The listing builds one solid part. Answer for the finished solid, in the listing's coordinates (mm). Give positions to 0.01 mm unless a question says otherwise; leave off trailing zeros. Order: outer loops, then holes, each group sorted by start corner. A loop starts at its lowest first (then second) coordinate and runs counter-clockwise, first axis right, second up. Notation, with made-up numbers: (38.5, 86.25) - (62.5, 86.25) arc R15 ccw to (62.5, 91.25) - close; hole circle Ø2 at (43, 23). An arc over 180 degrees is marked (long way). Use a Markdown table: item, result. Add a question column.
1) Flat-ended cylindrical pins translate along their axes: pin 1 (4 mm diameter, centred on x = 84, z = 6.8, fed in from +Y); pin 2 (4 mm diameter, centred on y = -81, z = 44, fed in from +X); pin 3 (1.2 mm diameter, centred on x = -38.5, y = -83, fed in from -Z). Find the tip coordinate at first contact, or state that the pin passes through.
2) Straight lines are drawn through the part: line 1 (X direction, y = -85, z = 20); line 2 (X direction, y = -90.1, z = 7); line 3 (X direction, y = -78.75, z = 31.5). For each, find the intervals that lie inside material, in ascending order.
3) Find section A-A, the plane x = -20. Determine the outline of the cut face in (y, z), plus the area to 3 significant figures.
4) Find section B-B, the plane z = 58.5. Determine the outline of the cut face in (x, y), plus the area to 3 significant figures.
from build123d import *

# Parameters (mm, degrees)
SKETCH006_R             = 4
SKETCH006_W             = 72
SKETCH006_H             = 15
SKETCH006_W_2           = 60
SKETCH006_H_2           = 8
PAD002_DEPTH            = 2.1
SKETCH010_R             = 1.6
POCKET004_DEPTH         = 5
SKETCH012_R             = 1.05
PAD004_DEPTH            = 11
SKETCH018_W             = 200
SKETCH018_H             = 5
PAD009_DEPTH            = 8
SKETCH019_W             = 31
SKETCH019_H             = 10
POCKET_DEPTH            = 5
SKETCH020_R             = 1.5
POCKET007_DEPTH         = 195
FILLET009_R             = 2.45
BODY002_PLACEMENT_ANGLE = 180


with BuildPart() as part:
    # Sketch006 → Pad002 (new body)
    with BuildSketch(Plane.XZ):
        with BuildLine():
            Line((-100, 0), (100, 0))
            ThreePointArc((101.6, -1.6), (101.131371, -0.468629), (100, 0))
            Line((101.6, -1.6), (101.6, -82.4))
            ThreePointArc((100, -84), (101.131371, -83.531371), (101.6, -82.4))
            Line((100, -89), (100, -84))
            Line((-100, -89), (100, -89))
            Line((-100, -84), (-100, -89))
            ThreePointArc((-101.6, -82.4), (-101.131371, -83.531371), (-100, -84))
            Line((-101.6, -1.6), (-101.6, -82.4))
            ThreePointArc((-100, 0), (-101.131371, -0.468629), (-101.6, -1.6))
        make_face()
        with Locations((-20, -70)):
            Circle(SKETCH006_R, mode=Mode.SUBTRACT)
        with Locations((20, -70)):
            Circle(SKETCH006_R, mode=Mode.SUBTRACT)
        with Locations((60, -70)):
            Circle(SKETCH006_R, mode=Mode.SUBTRACT)
        with Locations((-60, -70)):
            Circle(SKETCH006_R, mode=Mode.SUBTRACT)
        with Locations((0, -35.5)):
            Rectangle(SKETCH006_W, SKETCH006_H, mode=Mode.SUBTRACT)
        Polygon((-60.6, -14), (-60.6, -54), (-43, -54), (-43, -42), (-40, -14), align=None, mode=Mode.SUBTRACT)
        Polygon((40, -14), (60.6, -14), (60.6, -54), (43, -54), (43, -42), align=None, mode=Mode.SUBTRACT)
        with Locations((0, -18)):
            Rectangle(SKETCH006_W_2, SKETCH006_H_2, mode=Mode.SUBTRACT)
    extrude(amount=PAD002_DEPTH)

    # Sketch010 → Pocket004 (cut)
    with BuildSketch(Plane.XZ.offset(2.1)):
        with Locations((-84, -6.8)):
            Circle(SKETCH010_R)
        with Locations((84, -6.8)):
            Circle(SKETCH010_R)
        with Locations((94, -17)):
            Circle(SKETCH010_R)
        with Locations((94, -69)):
            Circle(SKETCH010_R)
        with Locations((-94, -69)):
            Circle(SKETCH010_R)
        with Locations((-94, -17)):
            Circle(SKETCH010_R)
        with Locations((0, -7)):
            Circle(SKETCH010_R)
        with Locations((-94, -43)):
            Circle(SKETCH010_R)
        with Locations((94, -43)):
            Circle(SKETCH010_R)
    extrude(amount=-POCKET004_DEPTH, mode=Mode.SUBTRACT)

    # Sketch012 → Pad004 (join)
    with BuildSketch(Plane.ZX):
        with BuildLine():
            Line((-52.5, 40), (-18.5, 40))
            ThreePointArc((-17.5, 39), (-17.792893, 39.707107), (-18.5, 40))
            Line((-17.5, 39), (-17.5, 36.5))
            ThreePointArc((-21.682412, 34.767588), (-19.012426, 34.236495), (-17.5, 36.5))
            Line((-21.682412, 34.767588), (-23, 36.085177))
            Line((-48, 36.085177), (-23, 36.085177))
            Line((-49.317588, 34.767588), (-48, 36.085177))
            ThreePointArc((-53.5, 36.5), (-51.987574, 34.236495), (-49.317588, 34.767588))
            Line((-53.5, 39), (-53.5, 36.5))
            ThreePointArc((-52.5, 40), (-53.207107, 39.707107), (-53.5, 39))
        make_face()
        with Locations((-20, 37.5)):
            Circle(SKETCH012_R, mode=Mode.SUBTRACT)
        with Locations((-51, 37.5)):
            Circle(SKETCH012_R, mode=Mode.SUBTRACT)
        with BuildLine():
            Line((-52.5, -40), (-18.5, -40))
            ThreePointArc((-18.5, -40), (-17.792893, -39.707107), (-17.5, -39))
            Line((-17.5, -39), (-17.5, -36.5))
            ThreePointArc((-17.5, -36.5), (-19.012426, -34.236495), (-21.682412, -34.767588))
            Line((-23, -36.085177), (-21.682412, -34.767588))
            Line((-48, -36.085177), (-23, -36.085177))
            Line((-49.317588, -34.767588), (-48, -36.085177))
            ThreePointArc((-49.317588, -34.767588), (-51.987574, -34.236495), (-53.5, -36.5))
            Line((-53.5, -39), (-53.5, -36.5))
            ThreePointArc((-53.5, -39), (-53.207107, -39.707107), (-52.5, -40))
        make_face()
        with Locations((-51, -37.5)):
            Circle(SKETCH012_R, mode=Mode.SUBTRACT)
        with Locations((-20, -37.5)):
            Circle(SKETCH012_R, mode=Mode.SUBTRACT)
    extrude(amount=PAD004_DEPTH)

    # Sketch018 (on Face4 of Pad004) → Pad009 (join)
    with BuildSketch(Plane(origin=(0, 0, 0), x_dir=(1, 0, 0), z_dir=(0, 1, 0))):
        with Locations((0, 86.5)):
            Rectangle(SKETCH018_W, SKETCH018_H)
    extrude(amount=PAD009_DEPTH)

    # Sketch019 (on Face74 of Pad009) → Pocket (cut)
    with BuildSketch(Plane(origin=(0, 0, -89), x_dir=(1, 0, 0), z_dir=(0, 0, -1))):
        with Locations((-59.5, -6)):
            Rectangle(SKETCH019_W, SKETCH019_H)
        with Locations((59.5, -6)):
            Rectangle(SKETCH019_W, SKETCH019_H)
    extrude(amount=-POCKET_DEPTH, mode=Mode.SUBTRACT)

    # Sketch020 (on Face62 of Pocket) → Pocket007 (cut)
    with BuildSketch(Plane(origin=(-100, 0, 0), x_dir=(0, 0, -1), z_dir=(-1, 0, 0))):
        with Locations((86.5, -5.5)):
            Circle(SKETCH020_R)
    extrude(amount=-POCKET007_DEPTH, mode=Mode.SUBTRACT)

    # Fillet009
    fillet009_edges = [part.edges().sort_by_distance(p)[0] for p in [
        (87.5, 8, -89),
        (87.5, 8, -84),
        (0, -2.1, -89),
        (0, 8, -89),
        (0, 8, -84),
        (-87.5, 8, -89),
        (-87.5, 8, -84),
    ]]
    fillet(fillet009_edges, radius=FILLET009_R)


with BuildPart() as part_1:
    # Body002 placement: moved
    add(part.part.moved(Location((0, -89.1, 0))).rotate(Axis((0, -89.1, 0), (0, 1, 0)), BODY002_PLACEMENT_ANGLE))


solid = part_1.part
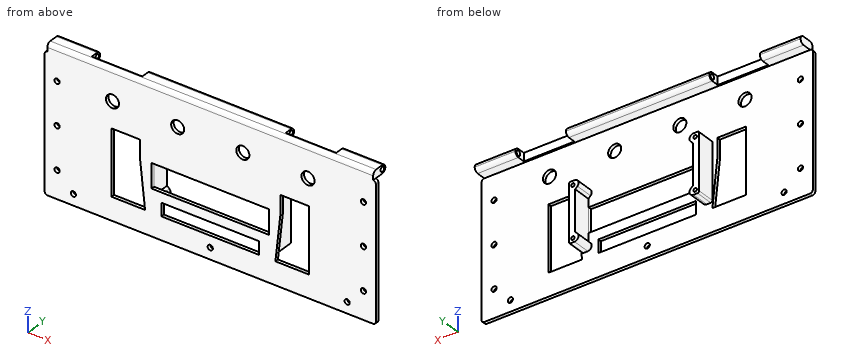
The answers:
| question | item | result |
|---|---|---|
| 1 | pin 1 | y = -89.1 |
| 1 | pin 2 | x = 40 |
| 1 | pin 3 | z = 17.5 |
| 2 | line 1 | -40 to -38.55, -36.45 to -34.05, 34.05 to 36.45, 38.55 to 40 |
| 2 | line 2 | -101.6 to -85.59, -82.41 to -1.6, 1.6 to 82.41, 85.59 to 101.6 |
| 2 | line 3 | -40 to -36.09, 36.09 to 40 |
| 3 | outline | (-91.2, 0) - (-89.1, 0) - (-89.1, 14) - (-91.2, 14) - close; (-91.2, 22) - (-89.1, 22) - (-89.1, 28) - (-91.2, 28) - close; (-91.2, 43) - (-89.1, 43) - (-89.1, 66) - (-91.2, 66) - close; (-91.2, 74) - (-89.1, 74) - (-89.1, 84) - (-83.55, 84) arc R2.45 ccw to (-81.1, 86.45) - (-81.1, 86.55) arc R2.45 ccw to (-83.55, 89) - (-88.75, 89) arc R2.45 ccw to (-91.2, 86.55) - close; hole circle Ø3 at (-83.6, 86.5) |
| 3 | area | 151 mm2 |
| 4 | outline | (-101.6, -91.2) - (101.6, -91.2) - (101.6, -89.1) - (-101.6, -89.1) - close |
| 4 | area | 427 mm2 |
